from build123d import *

# Parameters (mm, degrees)
SKETCH1_R           = 3.96875
BOSS_EXTRUDE1_DEPTH = 1.5875


with BuildPart() as part:
    # Sketch1 → Boss-Extrude1 (new body, symmetric)
    with BuildSketch(Plane.XY):
        with BuildLine():
            Line((0, 0), (0, -57.15))
            ThreePointArc((0, -57.15), (19.05, -76.2), (38.1, -57.15))
            Line((38.1, -57.15), (38.1, -31.75))
            Line((38.1, -31.75), (152.4, -31.75))
            Line((152.4, -31.75), (152.4, 0))
            Line((152.4, 0), (0, 0))
        make_face()
        with Locations((19.05, -57.15)):
            Circle(SKETCH1_R, mode=Mode.SUBTRACT)
    extrude(amount=BOSS_EXTRUDE1_DEPTH, both=True)


solid = part.part
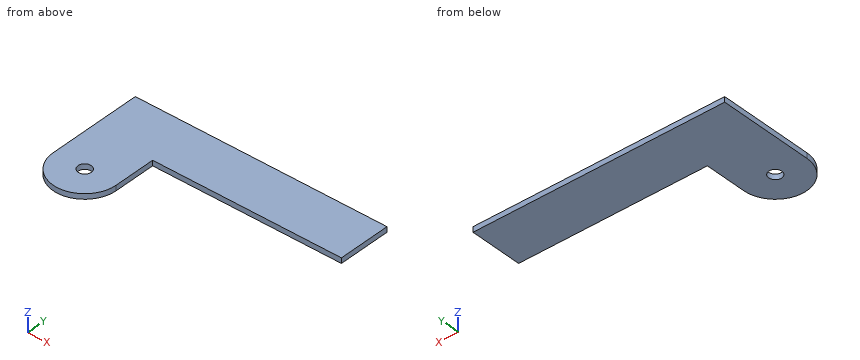
Design review of the part built by this model. Coordinates are the model's own, in mm. Round coordinates to 2 decimals unless told otherwise and drop trailing zeros. Order: outer loops, then holes, each group sorted by start corner. A loop starts at its lowest first (then second) coordinate and runs counter-clockwise, first axis right, second up. Notation, with made-up numbers: M 48,-36.5 L 66,-36.5 A22 cw 66,-7.5 Z; hole C 44,43 d4. An arc over 180 degrees is marked long. Answer as CSV lines item,"result". Start each with the question number.
1) Add section C-C (y = -41). Give the boundary of the cut face in (x, z), then the cut area to 3 significant figures.
2) Wall thickness on line 1 along Y through (x, z) = (19.05, 0.5); line 2 along Y through (x, z) = (108, 1.3); line 3 along X through (y, z) = (-36.5, -0.7): over which ranges is each line inside the solid? List them lowest first. Write a range as [from, to].
3) Add section B-B (z = 1.1). Give the boundary of the cut face in (x, y), then the cut area to 3 significant figures.
4) Add section A-A (x = 19.05). Give the boundary of the cut face in (y, z), then the cut area to 3 significant figures.
5) For pin 1 Ø1.6 at (y, z) = (-39, -0.5) entering from +X; pin 2 Ø1 at (y, z) = (-68, 0.5) entering from +X; pin 3 Ø10.5 at (x, y) = (19.05, -57.15) entering from -Z, all flat-tipped, find the tip position at first contact; note any pin that passes through.
6) Add section D-D (x = 140.5). Give the boundary of the cut face in (y, z), then the cut area to 3 significant figures.
Resolved:
1,outline,"M 0,-1.59 L 38.1,-1.59 L 38.1,1.59 L 0,1.59 Z"
1,area,"121 mm^2"
2,line 1,"[-76.2, -61.12], [-53.18, 0]"
2,line 2,"[-31.75, 0]"
2,line 3,"[0, 38.1]"
3,outline,"M 0,-57.15 A19.05 ccw 38.1,-57.15 L 38.1,-31.75 L 152.4,-31.75 L 152.4,0 L 0,0 Z; hole C 19.05,-57.15 d7.94"
3,area,"6,330 mm^2"
4,outline,"M -76.2,-1.59 L -61.12,-1.59 L -61.12,1.59 L -76.2,1.59 Z; M -53.18,-1.59 L 0,-1.59 L 0,1.59 L -53.18,1.59 Z"
4,area,"217 mm^2"
5,pin 1,"x = 38.1"
5,pin 2,"x = 35.04"
5,pin 3,"z = -1.59"
6,outline,"M -31.75,-1.59 L 0,-1.59 L 0,1.59 L -31.75,1.59 Z"
6,area,"101 mm^2"
